```python
from build123d import *

# Parameters (mm, degrees)
PAD042_DEPTH = 4.75


with BuildPart() as case1:
    # Sketch042 → Pad042 (new body)
    with BuildSketch(Plane.XY.offset(21.75)):
        with BuildLine():
            ThreePointArc((131.340316, 107.243249), (0, 110.109105), (-131.340316, 107.243249))
            ThreePointArc((-131.340316, 107.243249), (-138.945789, 104.356177), (-143.297313, 97.482848))
            ThreePointArc((-143.297313, 97.482848), (-155.054952, 0.033785), (-143.313373, -97.417215))
            ThreePointArc((-143.313373, -97.417215), (-138.877345, -104.411658), (-131.096658, -107.250934))
            ThreePointArc((-131.096658, -107.250934), (0, -110.106161), (131.096658, -107.250934))
            ThreePointArc((131.096658, -107.250934), (138.833073, -104.447134), (143.286208, -97.52738))
            ThreePointArc((143.286208, -97.52738), (155.054743, -0.079681), (143.324086, 97.372584))
            ThreePointArc((143.324086, 97.372584), (138.989661, 104.320204), (131.340316, 107.243249))
        make_face()
    extrude(amount=-PAD042_DEPTH)


with BuildPart() as case_bottom_plane:
    # Sketch040 → Loft002 section 0
    with BuildSketch(Plane.XY.offset(17)):
        with BuildLine():
            ThreePointArc((131.5, 112.710757), (0, 115.580098), (-131.5, 112.710757))
            ThreePointArc((-131.5, 112.710757), (-142.354422, 108.63407), (-148.591078, 98.859511))
            ThreePointArc((-148.591078, 98.859511), (-160.524221, 0.112742), (-148.644672, -98.640489))
            ThreePointArc((-148.644672, -98.640489), (-142.441793, -108.562815), (-131.5, -112.710757))
            ThreePointArc((-131.5, -112.710757), (0, -115.580098), (131.5, -112.710757))
            ThreePointArc((131.5, -112.710757), (142.354422, -108.63407), (148.591078, -98.859511))
            ThreePointArc((148.591078, -98.859511), (160.524221, -0.112742), (148.644672, 98.640489))
            ThreePointArc((148.644672, 98.640489), (142.441793, 108.562815), (131.5, 112.710757))
        make_face()
    # Sketch041 → Loft002 section 1
    with BuildSketch(Plane.XY.offset(25)):
        with BuildLine():
            ThreePointArc((131.340316, 107.243249), (0, 110.109105), (-131.340316, 107.243249))
            ThreePointArc((-131.340316, 107.243249), (-138.945789, 104.356177), (-143.297313, 97.482848))
            ThreePointArc((-143.297313, 97.482848), (-155.054952, 0.033785), (-143.313373, -97.417215))
            ThreePointArc((-143.313373, -97.417215), (-138.877345, -104.411658), (-131.096658, -107.250934))
            ThreePointArc((-131.096658, -107.250934), (0, -110.106161), (131.096658, -107.250934))
            ThreePointArc((131.096658, -107.250934), (138.833073, -104.447134), (143.286208, -97.52738))
            ThreePointArc((143.286208, -97.52738), (155.054743, -0.079681), (143.324086, 97.372584))
            ThreePointArc((143.324086, 97.372584), (138.989661, 104.320204), (131.340316, 107.243249))
        make_face()
    loft()

    # Cut002: cut CASE1
    add(case1.part, mode=Mode.SUBTRACT)


solid = case_bottom_plane.part
```
Can you work these out from the model? Positions are in its coordinate system, mm. A direction names the side the tool comes from. Give positions to 0.01 mm unless a question says otherwise; leave off trailing zeros. One line per question, with ' | ' between items. Start each with the question number.
Q1. If I drill on line 1 (Z direction, x = -53.5, y = -0.5); line 2 (X direction, y = -80.5, z = 20); line 3 (X direction, y = 104.5, z = 20.75), over which ranges is the centre line in solid material (lowest first)? Write a range as from..to.
Q2. For faces 1 (the flat face through (-8, 114, 17)), 2 (the cylindrical face through (-138.856, 104.429, 19.408)), which set-ups out of +Z, -Z, +X, -X, +Y, -Y let a thin tool reach every point of the face, with its end or its side?
Q3. If we mould it in two halves opening along Y, with no side actions, what happens to faces 3 (the flat face through (-2, -1, 25)), 4 (the cylindrical face through (-138.969, -104.337, 19.408))? For each: +Y half, -Y half, draft (parallel to the pull), parting line (faces both ways), or undercut.
Q4. For pin 1 Ø6 at (x, y) = (-91, 2) entering from -Z; pin 2 Ø1.5 at (y, z) = (-26, 20.5) entering from +X; pin 3 Ø1.5 at (x, z) = (-120, 18.5) entering from +Y, each with a flat end and sliding along its axis, tell me the tip position at first contact or that it passes through.
Computed:
1) line 1: z = 21.75..25 | line 2: x = -150.56..-147.07, 147.07..150.56 | line 3: x = -142.91..-138.77, 138.77..142.91
2) face 1: -Z, +X, -X, +Y, -Y | face 2: -Z
3) face 3: draft | face 4: undercut
4) pin 1: stops at z = 21.75 | pin 2: stops at x = 157.83 | pin 3: stops at y = 112.68
